Build history of the part. All positions in model axes, mm. Give positions to 0.01 mm unless a question says otherwise; leave off trailing zeros. Write each loop counter-clockwise with the first axis right and the second up, starting at its lowest first coordinate (ties: lowest second). Pieces come first, ordered by that corner, then holes. Notation, with made-up numbers: M -28,22.25 L 22,22.25 A25 ccw 22,42.25 Z; hole C -31,-38 d11. An arc over 180 degrees is marked long. One line per item, written item: value. Start each with the question number.
from build123d import *

# Parameters (mm, degrees)
SKETCH3_R          = 1.174710487
CUT_EXTRUDE1_DEPTH = 0.2
CHAMFER1_SIZE      = 1


with BuildPart() as part:
    # Sketch2 → Revolve1 (revolve)
    with BuildSketch(Plane.XY):
        with BuildLine():
            Line((28.5, 0), (39, 0))
            Line((39, 0), (39, 4.75))
            Line((39, 4.75), (34.117811535, 4.75))
            ThreePointArc((34.117811535, 4.75), (31.774779013, 4.167788181), (29.431746492, 4.75))
            Line((29.431746492, 4.75), (28.5, 4.75))
            Line((28.5, 4.75), (28.5, 0))
        make_face()
    revolve(axis=Axis((0, 0, 0), (0, 1, 0)))

    # Sketch3 → Cut-Extrude1 (cut)
    with BuildSketch(Plane(origin=(0, 4.75, 0), x_dir=(1, 0, 0), z_dir=(0, 1, 0))):
        with Locations((38.381757848, 0)):
            Circle(SKETCH3_R)
    extrude(amount=-CUT_EXTRUDE1_DEPTH, mode=Mode.SUBTRACT)

    # Chamfer1
    chamfer1_edges = [part.edges().sort_by_distance(p)[0] for p in [
        (-39, 0, 0),
        (-28.5, 0, 0),
    ]]
    chamfer(chamfer1_edges, length=CHAMFER1_SIZE)


solid = part.part
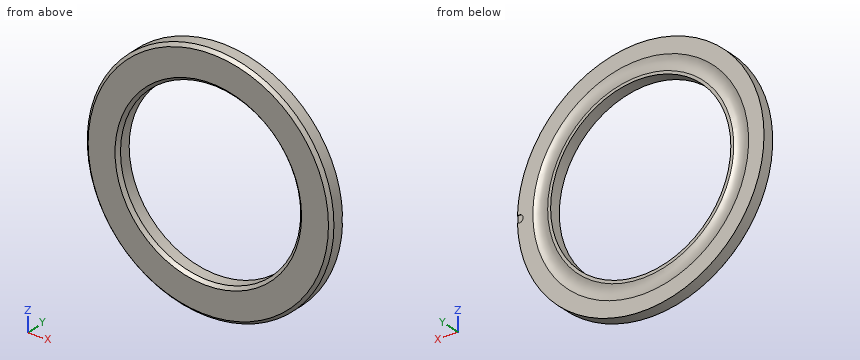
1) Drop flat-ended pins along their axis: P1, Ø1.5, axis at y = 3.5, z = -29, coming from the -X side; P2, Ø1.4, axis at x = 38.38, z = 0, coming from the +Y side. Give the stop position or say it passes through.
2) Band-saw the part on C-C (y = 2.25). List the corners of the cut face in (x, z), then the cut area to 3 significant figures.
3) Band-saw the part on A-A (z = 0). List the corners of the cut face in (x, y).
4) Band-saw the part on B-B (x = 0). List the corners of the cut face in (y, z).
5) Probe line 1 along Z through (x, y) = (0, 2.2); line 2 along X through (y, z) = (4.6, 0). List the from-to ranges inside material, lowest first. Write a range as from..to.
Model answer:
1. P1: stops at x = -26.89
1. P2: stops at y = 4.55
2. outline: C 0,0 d78; hole C 0,0 d57
2. area: 2,230 mm²
3. outline: M -39,1 L -38,0 L -29.5,0 L -28.5,1 L -28.5,4.75 L -29.43,4.75 A5.01 cw -34.12,4.75 L -39,4.75 Z; M 28.5,1 L 29.5,0 L 38,0 L 39,1 L 39,4.55 L 37.21,4.55 L 37.21,4.75 L 34.12,4.75 A5.01 cw 29.43,4.75 L 28.5,4.75 Z
4. outline: M 0,-38 L 1,-39 L 4.75,-39 L 4.75,-34.12 A5.01 cw 4.75,-29.43 L 4.75,-28.5 L 1,-28.5 L 0,-29.5 Z; M 0,29.5 L 1,28.5 L 4.75,28.5 L 4.75,29.43 A5.01 cw 4.75,34.12 L 4.75,39 L 1,39 L 0,38 Z
5. line 1: z = -39..-28.5, 28.5..39
5. line 2: x = -39..-33.81, -29.74..-28.5, 28.5..29.74, 33.81..37.21
